For this review, use the dimensioned drawing (mm, ordinates from the lowest corner) and the shaded views. Give positions to 0.01 mm unless a question says otherwise; leave off trailing zeros. Order: outer loops, then holes, each group sorted by start corner. A loop starts at its lowest first (then second) coordinate and runs counter-clockwise, first axis right, second up.
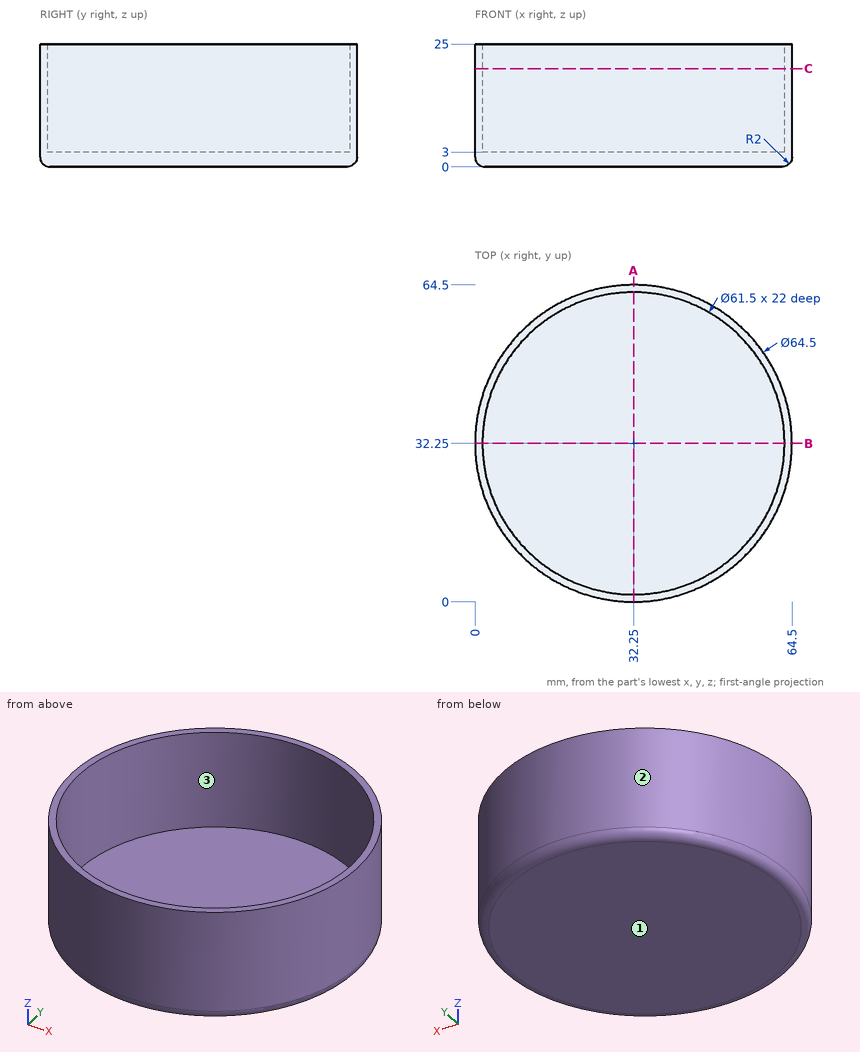
1. For line 1 along Y through (x, z) = (32.25, 11.25); line 2 along Z through (x, y) = (4, 42); line 3 along Y through (x, z) = (34, 13.5), list the stretches that pass through material, from the lowest coordinate up.
Recorded:
line 1: y = 0 to 1.5, 63 to 64.5
line 2: z = 0 to 3
line 3: y = 0.05 to 1.55, 62.95 to 64.45
2. For pin 1 (10 mm diameter, centred on y = 25.5, z = 17, fed in from +X); pin 2 (10 mm diameter, centred on y = 17.5, z = 17, fed in from +X); pin 3 (1.5 mm diameter, centred on y = 25.5, z = 22, fed in from -X), all flat-tipped, find the tip position at first contact; note any pin that passes through.
Recorded:
pin 1: stops at x = 64.45
pin 2: stops at x = 62.99
pin 3: stops at x = 0.56
3. Take a section at A-A (x = 32.25). State the section outline as (y, z) points.
Recorded:
outline: (0, 2) arc R2 ccw to (2, 0) - (62.5, 0) arc R2 ccw to (64.5, 2) - (64.5, 25) - (63, 25) - (63, 3) - (1.5, 3) - (1.5, 25) - (0, 25) - close
4. Draft analysis for pull direction X (two halves, no side actions). For the marked faces 1, 2 and 3, state which applies: pulls with the +X half, pulls with the -X half, needs draft (parallel to the pull), parting line crosses it, or undercut.
Recorded:
face 1: needs draft
face 2: parting line crosses it
face 3: undercut
5. Take a section at C-C (z = 20). State the section outline as (x, y) points, then the cut area to 3 significant figures.
Recorded:
outline: circle Ø64.5 at (32.25, 32.25); hole circle Ø61.5 at (32.25, 32.25)
area: 297 mm2
